Input: dimensioned drawing with shaded views. Units: mm. Origin: part minimum x, y, z. A direction names the side the tool comes from. Round coordinates to 2 decimals unless told otherwise and drop trailing zeros. Loops run counter-clockwise (first coordinate to the right, second up) from the corner with the lowest first, then second, coordinate; pieces in that order, holes last. Notation, with made-up numbers: M -10,84.25 L 49,84.25 A18 cw 49,102.25 Z; hole C -39,21 d3. An arc over 180 degrees is marked long. Return JSON: item names as keys, results as strings.
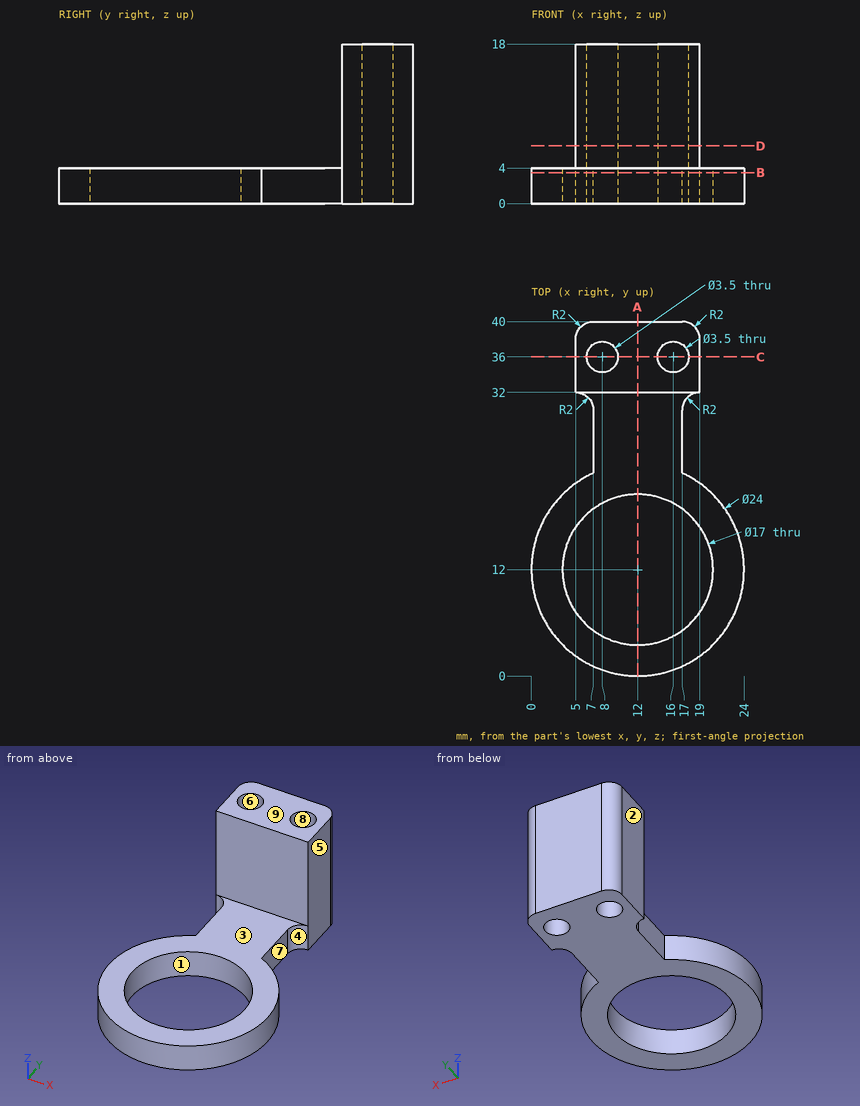
Q1. Pull-direction query (X, two-part tool) for the marked faces 6, 7, 8 and 9; classes: pulls with the +X half, pulls with the -X half, needs draft (parallel to the pull), parting line crosses it, or undercut.
Determined:
{"face 6": "undercut", "face 7": "pulls with the +X half", "face 8": "undercut", "face 9": "needs draft"}
Q2. Section query D-D (z = 6.5). Output: boundary loops of the cut face in (x, y).
Determined:
{"outline": "M 5,32 L 19,32 L 19,38 A2 ccw 17,40 L 7,40 A2 ccw 5,38 Z; hole C 8,36 d3.5; hole C 16,36 d3.5"}
Q3. Material intervals for L1, parallel to Y at x = 16, z = 12.5; L2, parallel to Y at x = 12, z = 2.95; L3, parallel to Z at x = 14, y = 25, sorted ascending.
Determined:
{"L1": "y = 32 to 34.25, 37.75 to 40", "L2": "y = 0 to 3.5, 20.5 to 40", "L3": "z = 0 to 4"}
Q4. Section query A-A (x = 12). Output: boundary loops of the cut face in (y, z), plus the area to 3 significant figures.
Determined:
{"outline": "M 0,0 L 3.5,0 L 3.5,4 L 0,4 Z; M 20.5,0 L 40,0 L 40,18 L 32,18 L 32,4 L 20.5,4 Z", "area": "204 mm^2"}
Q5. Section query B-B (z = 3.5). State how many separate pieces and enclosed holes the cut face has, plus the area to 3 significant figures.
Determined:
{"separate pieces": "1", "enclosed holes": "3", "area": "402 mm^2"}
Q6. Reachability of the marked faces 1, 2, 3, 4 and 5 from +Z, -Z, +X, -X, +Y, -Y: full face, straight path, thin tool, end or side. Return the list, or none.
Determined:
{"face 1": "+Z, -Z", "face 2": "+Z, -Z, -X, +Y", "face 3": "+Z, +X, -X, -Y", "face 4": "+Z, -Z, +X", "face 5": "+Z, -Z, +X, +Y"}
Q7. Section query C-C (y = 36). Output: boundary loops of the cut face in (x, z), plus the area to 3 significant figures.
Determined:
{"outline": "M 5,0 L 6.25,0 L 6.25,18 L 5,18 Z; M 9.75,0 L 14.25,0 L 14.25,18 L 9.75,18 Z; M 17.75,0 L 19,0 L 19,18 L 17.75,18 Z", "area": "126 mm^2"}
Q8. Pin query (flat end, axial travel): pin 1 (3 mm diameter, centred on x = 16, y = 36, fed in from -Z); pin 2 (3 mm diameter, centred on y = 27, z = 3, fed in from +X); pin 3 (7 mm diameter, centred on x = 12.5, z = 10.5, fed in from -Y); pin 4 (7 mm diameter, centred on x = 16.5, y = 18, fed in from +Z). Return the tip coordinate at first contact, or that it passes through.
Determined:
{"pin 1": "passes through", "pin 2": "stops at x = 17", "pin 3": "stops at y = 32", "pin 4": "stops at z = 4"}
